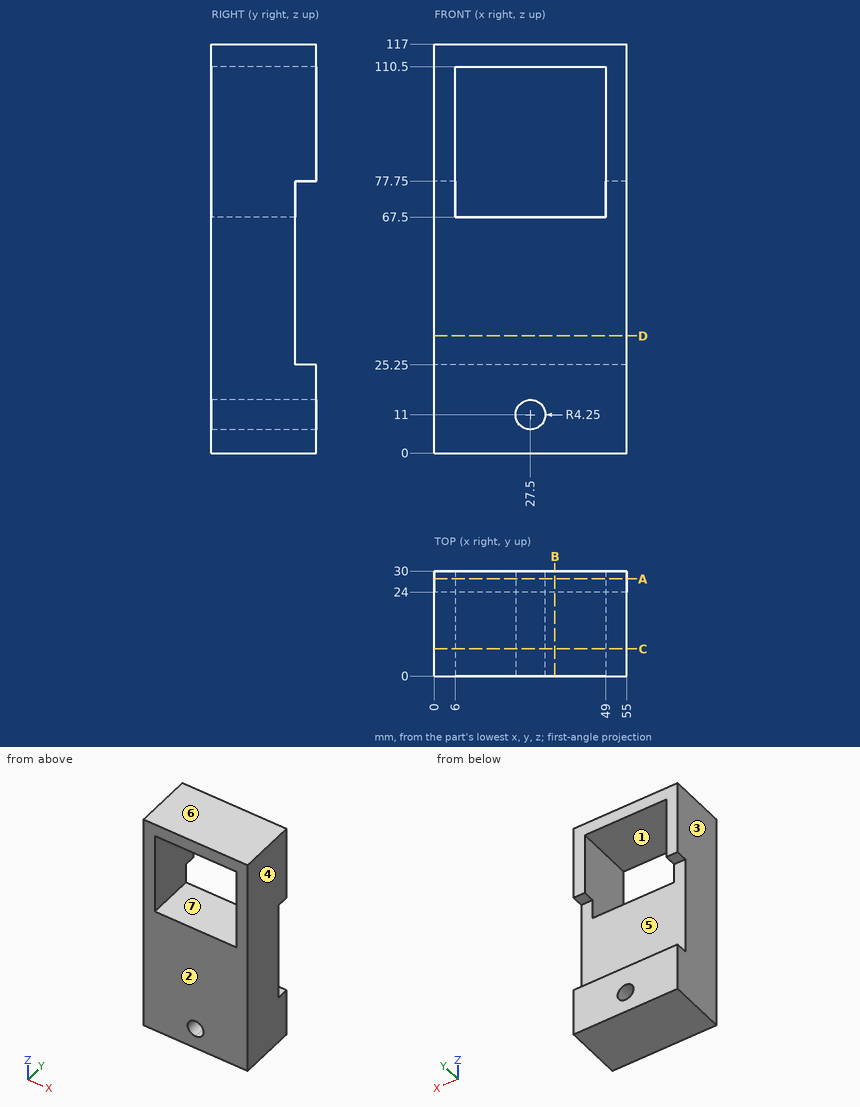
Job drawing, mm, ordinate dimensions from the low corner. One solid piece. A direction names the side the tool comes from. Coordinates: 2 decimals unless noted, no trailing zeros. Order: outer loops, then holes, each group sorted by start corner. A loop starts at its lowest first (then second) coordinate and runs counter-clockwise, first axis right, second up. Notation, with made-up numbers: (8, -35.75) -> (35, -35.75) arc R7 ccw to (35, -24.75) -> close; hole circle Ø6 at (15.5, -28.5). An arc over 180 degrees is marked (long way). Answer in a Markdown table with one row per item. Add a question column.
Q1. Which spindle directions (+Z, -Z, +X, -X, +Y, -Y) get a long thin tool onto all of the face, cutting with end or side? Do the marked faces 5, 6 and 7. Say none if no direction does.
Q2. Mould opens along X. For the marked faces 1, 2, 3 and 4 say: +X half, -X half, draft (parallel to the pull), parting line (faces both ways), or undercut.
Q3. Band-saw the part on A-A, the plane y = 27.75. List the corners of the cut face in (x, z).
Q4. Band-saw the part on C-C, the plane y = 7.75. List the corners of the cut face in (x, z).
Q5. Band-saw the part on D-D, the plane z = 33.5. List the corners of the cut face in (x, y), then the cut area to 3 significant figures.
Q6. Wall check: line 1 along Z through (x, y) = (27.5, 19.5); line 2 along X through (y, z) = (25.75, 87.5); line 3 along Z through (x, y) = (21, 19.25). Give the ranges that are in metal, low to high. Write a range as [from, to].
Q7. Drop a flat-ended pin along its axis: pin 1 (5 mm diameter, centred on x = 43.5, z = 36.5, fed in from +Y). Give the stop position or say it passes through.
Q8. Band-saw the part on B-B, the plane x = 34.5. List the corners of the cut face in (y, z).
Answers follow:
| question | item | result |
|---|---|---|
| 1 | face 5 | +X, -X, +Y |
| 1 | face 6 | +Z, +X, -X, +Y, -Y |
| 1 | face 7 | +Y, -Y |
| 2 | face 1 | undercut |
| 2 | face 2 | draft |
| 2 | face 3 | -X half |
| 2 | face 4 | +X half |
| 3 | outline | (0, 0) -> (55, 0) -> (55, 25.25) -> (0, 25.25) -> close; (0, 77.75) -> (6, 77.75) -> (6, 110.5) -> (49, 110.5) -> (49, 77.75) -> (55, 77.75) -> (55, 117) -> (0, 117) -> close; hole (23.25, 11) arc R4.25 ccw (long way) to (27.5, 15.25) arc R4.25 ccw to start |
| 4 | outline | (0, 0) -> (55, 0) -> (55, 117) -> (0, 117) -> close; hole (6, 67.5) -> (49, 67.5) -> (49, 110.5) -> (6, 110.5) -> close; hole (23.25, 11) arc R4.25 ccw (long way) to (27.5, 15.25) arc R4.25 ccw to start |
| 5 | outline | (0, 0) -> (55, 0) -> (55, 24) -> (0, 24) -> close |
| 5 | area | 1,320 mm^2 |
| 6 | line 1 | [0, 6.75], [15.25, 67.5], [110.5, 117] |
| 6 | line 2 | [0, 6], [49, 55] |
| 6 | line 3 | [0, 67.5], [110.5, 117] |
| 7 | pin 1 | y = 24 |
| 8 | outline | (0, 0) -> (30, 0) -> (30, 25.25) -> (24, 25.25) -> (24, 67.5) -> (0, 67.5) -> close; (0, 110.5) -> (30, 110.5) -> (30, 117) -> (0, 117) -> close |
